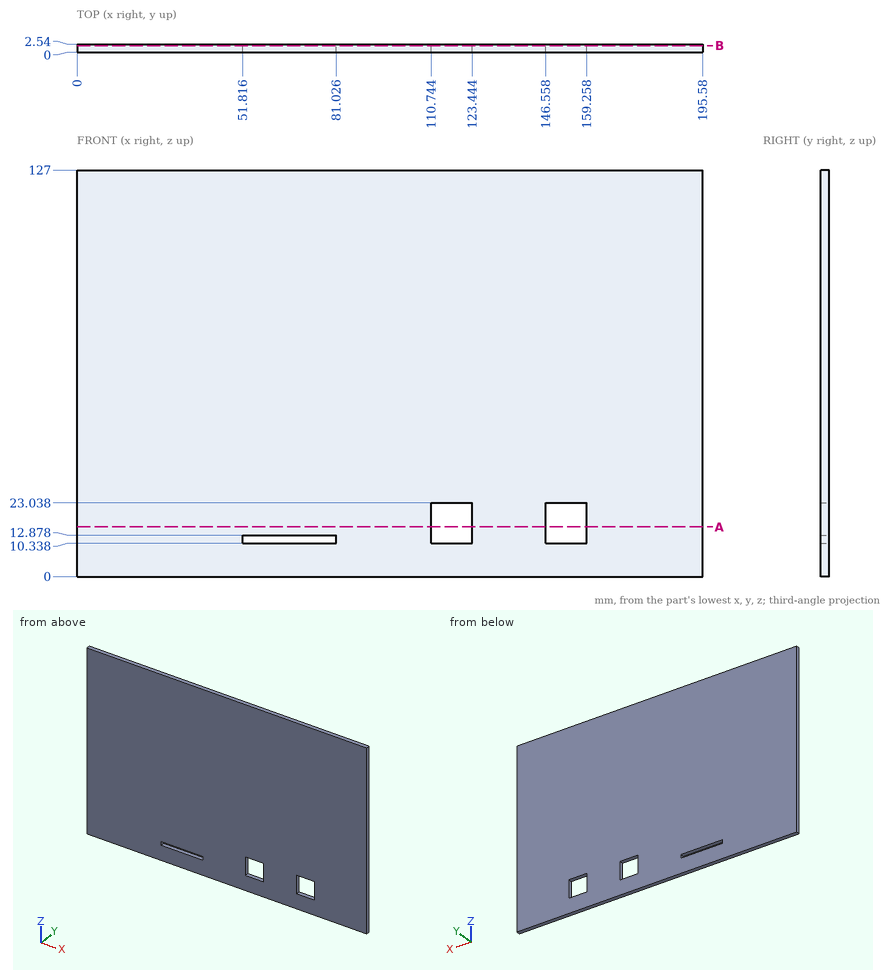
Verification items for this drawing (mm, ordinates from the low corner). Coordinates: 2 decimals unless noted, no trailing zeros. Order: outer loops, then holes, each group sorted by start corner. A loop starts at its lowest first (then second) coordinate and runs counter-clockwise, first axis right, second up. Notation, with made-up numbers: (72.25, 47.5) - (105.25, 47.5) arc R32 ccw to (105.25, 82.5) - close; hole circle Ø11 at (0, 27). An arc over 180 degrees is marked (long way). Answer in a Markdown table with one row per item. Add a question column.
1. Section check B-B (y = 2.05). Enter the section's corners in (x, z).
2. Section check A-A (z = 15.5). Enter the section's corners in (x, y).
3. Material ranges on L1, parallel to X at y = 1, z = 21; L2, parallel to Z at x = 77, y = 1.65; L3, parallel to Z at x = 116, y = 1, recorded low to high. Write a range as [from, to].
Data:
| question | item | result |
|---|---|---|
| 1 | outline | (0, 0) - (195.58, 0) - (195.58, 127) - (0, 127) - close; hole (51.82, 10.34) - (81.03, 10.34) - (81.03, 12.88) - (51.82, 12.88) - close; hole (110.74, 10.34) - (123.44, 10.34) - (123.44, 23.04) - (110.74, 23.04) - close; hole (146.56, 10.34) - (159.26, 10.34) - (159.26, 23.04) - (146.56, 23.04) - close |
| 2 | outline | (0, 0) - (110.74, 0) - (110.74, 2.54) - (0, 2.54) - close; (123.44, 0) - (146.56, 0) - (146.56, 2.54) - (123.44, 2.54) - close; (159.26, 0) - (195.58, 0) - (195.58, 2.54) - (159.26, 2.54) - close |
| 3 | L1 | x = [0, 110.74], [123.44, 146.56], [159.26, 195.58] |
| 3 | L2 | z = [0, 10.34], [12.88, 127] |
| 3 | L3 | z = [0, 10.34], [23.04, 127] |
